Here's how the part is built. I have some questions about the finished solid (model axes, mm). A direction names the side the tool comes from. Round coordinates to 2 decimals unless told otherwise and drop trailing zeros. Loops run counter-clockwise (first coordinate to the right, second up) from the corner with the lowest first, then second, coordinate; pieces in that order, holes last. Notation, with made-up numbers: (-37.75, 56.5) - (20.25, 56.5) arc R18 cw to (20.25, 69.5) - close; hole circle Ø8 at (15.25, -17). An arc over 180 degrees is marked (long way). Answer as a JSON object with one key per item and string values. Group by question number.
1) Will these pins go through, and if not, where does the flat tip stop? P1, Ø2, axis at x = 3, z = -3.5, coming from the -Y side; P2, Ø1.5, axis at y = 1, z = 3.5, coming from the +X side.
2) I want a section at B-B, the plane z = -2.25. Please give me the cut outline in (x, y) (1 decimal), then the cut area to 3 significant figures.
3) Which directions (+Z, -Z, +X, -X, +Y, -Y) give clear straight access to the entire face, cutting with the end or side of a thin tool? Please do faces 1 (the face through (0, -7, 0)), 2 (the face through (0, 5, -1.588)), 3 (the face through (-2, 2, 7.588)).
4) If I drill on line 1 along Z through (x, y) = (-1, -7); line 2 along Y through (x, z) = (0, 4); line 3 along X through (y, z) = (0, -0.25), over which ranges is the centre line in solid material (lowest first)? Write a range as [from, to].
5) I want a section at A-A, the plane y = -2. Please give me the cut outline in (x, z), then the cut area to 3 significant figures.
6) If we mould it in two halves opening along X, with no side actions, what happens to faces 4 (the face through (-1.72, -7.75, 6.78)), 5 (the face through (2.385, -0.751, -0.284)), 6 (the face through (2, 2, -7.938))? For each: pulls with the +X half, pulls with the -X half, needs draft (parallel to the pull), parting line crosses it, or undercut.
7) I want a section at D-D, the plane x = -2.75. Please give me the cut outline in (y, z).
8) I want a section at C-C, the plane x = 1. Please give me the cut outline in (y, z), then the cut area to 3 significant figures.
from build123d import *

# Parameters (mm, degrees)
F0_R         = 6.35
F1_DEPTH     = 6
F2_R         = 7.9375
F3_DEPTH     = 1.5875
F4_R         = 7.9375
F5_DEPTH     = 1.5875
F6_W         = 9.525
F6_H         = 9.525
F7_DEPTH     = 6.35
F8_R         = 2.5
F9_DEPTH     = 15.525
F11_REACH    = 16.5631366107
F12_T1_DEPTH = 18.25625


# Not quite as in the source:
# - a fillet or chamfer that OpenCascade refuses, or shapes differently, is made with other operations: its cross-section is extruded or revolved along the edge and cut away or added


with BuildPart() as f1:
    # F0 (on Top) → F1 (new body)
    with BuildSketch(Plane.XY):
        Circle(F0_R)
    extrude(amount=F1_DEPTH)

    # F2 (on face) → F3 (join)
    with BuildSketch(Plane.XY.offset(6)):
        Circle(F2_R)
    extrude(amount=F3_DEPTH)

    # F4 (on face) → F5 (join)
    with BuildSketch(Plane(origin=(0, 0, 0), x_dir=(1, 0, 0), z_dir=(0, 0, -1))):
        Circle(F4_R)
    extrude(amount=F5_DEPTH)

    # F6 (on face) → F7 (join)
    with BuildSketch(Plane(origin=(0, 0, -1.5875), x_dir=(1, 0, 0), z_dir=(0, 0, -1))):
        Rectangle(F6_W, F6_H)
    extrude(amount=F7_DEPTH)

    # F8 (on face) → F9 (cut, through all)
    with BuildSketch(Plane(origin=(0, 0, -7.9375), x_dir=(1, 0, 0), z_dir=(0, 0, -1))):
        Circle(F8_R)
    extrude(amount=-F9_DEPTH, mode=Mode.SUBTRACT)

    f11_end = f1.faces().sort_by_distance((-2.5, 0, -0.175))[0]
    # F10 (on face) → F11 (cut, up to a face of the model that its end follows)
    with BuildSketch(Plane(origin=(-4.7625, 0, 0), x_dir=(0, -1, 0), z_dir=(-1, 0, 0))):
        with BuildLine():
            ThreePointArc((0, -3.0353), (-1.7272, -4.7625), (0, -6.4897))
            Line((0, -6.4897), (0, -3.0353))
        make_face()
        with BuildLine():
            Line((0, -3.0353), (0, -6.4897))
            ThreePointArc((0, -6.4897), (1.2213148325, -5.9838148325), (1.7272, -4.7625))
            ThreePointArc((1.7272, -4.7625), (1.2213148325, -3.5411851675), (0, -3.0353))
        make_face()
    f11_long = extrude(amount=-F11_REACH, mode=Mode.PRIVATE)
    add(split(f11_long, bisect_by=f11_end, keep=Keep.ALL, mode=Mode.PRIVATE).solids().sort_by_distance((-4.7625, 0, -4.7625))[0], mode=Mode.SUBTRACT)

    # F12: fillet of radius 4.7625 on 4 edges, made by hand

    # F12_s2 → F12_t1 (cut)
    with BuildSketch(Plane.XY.offset(-19.84375)):
        with BuildLine():
            ThreePointArc((-4.7625, 0), (-3.3675960454, -3.3675960454), (0, -4.7625))
            Line((0, -4.7625), (-4.7625, -4.7625))
            Line((-4.7625, -4.7625), (-4.7625, 0))
        make_face()
        with BuildLine():
            ThreePointArc((-4.7625, 0), (-3.3675960454, 3.3675960454), (0, 4.7625))
            Line((0, 4.7625), (-4.7625, 4.7625))
            Line((-4.7625, 4.7625), (-4.7625, 0))
        make_face()
        with BuildLine():
            ThreePointArc((0, 4.7625), (3.3675960454, 3.3675960454), (4.7625, 0))
            Line((4.7625, 0), (4.7625, 4.7625))
            Line((4.7625, 4.7625), (0, 4.7625))
        make_face()
        with BuildLine():
            ThreePointArc((4.7625, 0), (3.3675960454, -3.3675960454), (0, -4.7625))
            Line((0, -4.7625), (4.7625, -4.7625))
            Line((4.7625, -4.7625), (4.7625, 0))
        make_face()
    extrude(amount=F12_T1_DEPTH, mode=Mode.SUBTRACT)


solid = f1.part
Outcome:
{
 "1": {"P1": "y = -4.32", "P2": "x = 6.35"},
 "2": {"outline": "circle Ø9.5 at (0, 0); hole circle Ø5 at (0, 0)", "area": "51.6 mm^2"},
 "3": {"face 1": "none", "face 2": "-Z", "face 3": "+Z, +X, -X, +Y, -Y"},
 "4": {"line 1": "[-1.59, 0], [6, 7.59]", "line 2": "[-6.35, -2.5], [2.5, 6.35]", "line 3": "[-7.94, -2.5], [2.5, 7.94]"},
 "5": {"outline": "(-7.68, -1.59) - (-4.32, -1.59) - (-4.32, -7.94) - (-1.5, -7.94) - (-1.5, 7.59) - (-7.68, 7.59) - (-7.68, 6) - (-6.03, 6) - (-6.03, 0) - (-7.68, 0) - close; (1.5, -7.94) - (4.32, -7.94) - (4.32, -1.59) - (7.68, -1.59) - (7.68, 0) - (6.03, 0) - (6.03, 6) - (7.68, 6) - (7.68, 7.59) - (1.5, 7.59) - close", "area": "129 mm^2"},
 "6": {"face 4": "parting line crosses it", "face 5": "undercut", "face 6": "needs draft"},
 "7": {"outline": "(-7.45, -1.59) - (-3.89, -1.59) - (-3.89, -7.94) - (3.89, -7.94) - (3.89, -1.59) - (7.45, -1.59) - (7.45, 0) - (5.72, 0) - (5.72, 6) - (7.45, 6) - (7.45, 7.59) - (-7.45, 7.59) - (-7.45, 6) - (-5.72, 6) - (-5.72, 0) - (-7.45, 0) - close; hole circle Ø3.45 at (0, -4.76)"},
 "8": {"outline": "(-7.87, -1.59) - (-4.66, -1.59) - (-4.66, -7.94) - (-2.29, -7.94) - (-2.29, 7.59) - (-7.87, 7.59) - (-7.87, 6) - (-6.27, 6) - (-6.27, 0) - (-7.87, 0) - close; (2.29, -7.94) - (4.66, -7.94) - (4.66, -1.59) - (7.87, -1.59) - (7.87, 0) - (6.27, 0) - (6.27, 6) - (7.87, 6) - (7.87, 7.59) - (2.29, 7.59) - close", "area": "113 mm^2"}
}
